Answer from the drawing. Dimensions are ordinates in mm from the lowest x, y and z of the part. A direction names the side the tool comes from. Give positions to 0.01 mm unless a question says otherwise; leave off trailing zeros. Order: outer loops, then holes, each group sorted by start corner. A loop starts at its lowest first (then second) coordinate and runs counter-clockwise, first axis right, second up. Notation, with made-up numbers: (63.5, 2.5) - (109.5, 2.5) arc R20 ccw to (109.5, 27.5) - close; hole circle Ø3 at (17.5, 22). An arc over 180 degrees is marked (long way). Use a Markdown table: item, result. Add a question column.
1) For the marked faces 4, 5 and 6, determine the directions among +Z, -Z, +X, -X, +Y, -Y from which every point of the face is accessible in a straight line to the end or side of a thin tool.
2) Find section B-B, the plane y = 11.25. State how many separate pieces and enclosed holes the cut face has, plus the area to 3 significant figures.
3) Flat-ended cylindrical pins translate along their axes: pin 1 (10 mm diameter, centred on y = 5, z = 12.5, fed in from -X); pin 2 (3 mm diameter, centred on x = 35, y = 5, fed in from +Z); pin 3 (4.5 mm diameter, centred on x = 35, y = 10, fed in from +Z); pin 4 (10 mm diameter, centred on x = 33, y = 14, fed in from +Z). Find the tip coordinate at first contact, or state that the pin passes through.
4) Straight lines are drawn through the part: line 1 (Y direction, x = 35, z = 3.1); line 2 (Z direction, x = 7.5, y = 2.5); line 3 (Z direction, x = 20, y = 10.25). For each, find the intervals that lie inside material, in ascending order.
5) The mould has two halves that part along Y. Classify the marked faces 1, 2 and 3: released by +Y, released by -Y, zero draft, split by the parting line, or undercut.
6) Find section A-A, the plane x = 35. Determine the outline of the cut face in (y, z).
7) Find section D-D, the plane x = 9. Determine the outline of the cut face in (y, z).
8) Find section C-C, the plane z = 9. Determine the outline of the cut face in (x, y).
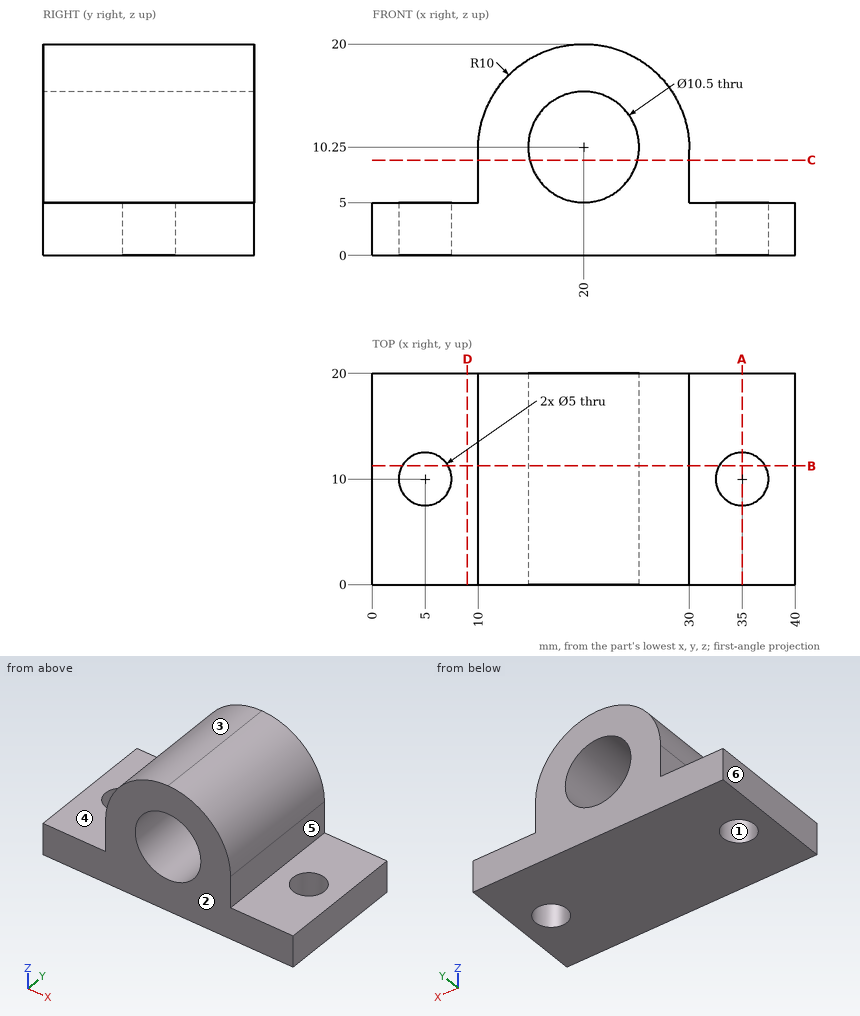
The answers:
| question | item | result |
|---|---|---|
| 1 | face 4 | +Z, -X, +Y, -Y |
| 1 | face 5 | +Z, +X, +Y, -Y |
| 1 | face 6 | +Z, -Z, -X, +Y, -Y |
| 2 | separate pieces | 3 |
| 2 | enclosed holes | 1 |
| 2 | area | 327 mm2 |
| 3 | pin 1 | x = 10 |
| 3 | pin 2 | z = 5 |
| 3 | pin 3 | through |
| 3 | pin 4 | z = 16 |
| 4 | line 1 | 0 to 7.5, 12.5 to 20 |
| 4 | line 2 | 0 to 5 |
| 4 | line 3 | 0 to 5, 15.5 to 20 |
| 5 | face 1 | undercut |
| 5 | face 2 | released by -Y |
| 5 | face 3 | zero draft |
| 6 | outline | (0, 0) - (7.5, 0) - (7.5, 5) - (0, 5) - close; (12.5, 0) - (20, 0) - (20, 5) - (12.5, 5) - close |
| 7 | outline | (0, 0) - (20, 0) - (20, 5) - (0, 5) - close |
| 8 | outline | (10, 0) - (14.9, 0) - (14.9, 20) - (10, 20) - close; (25.1, 0) - (30, 0) - (30, 20) - (25.1, 20) - close |
